```python
from build123d import *

# Parameters (mm, degrees)
F0_W     = 77.216
F0_H     = 148.336
F1_DEPTH = 14.478
F2_R     = 5.08
F3_T     = -6.858
F4_R     = 5.08


with BuildPart() as f1:
    # F0 (on Top) → F1 (new body)
    with BuildSketch(Plane.XY):
        Rectangle(F0_W, F0_H)
    extrude(amount=F1_DEPTH)

    # F2
    f2_edges = [f1.edges().sort_by_distance(p)[0] for p in [
        (-38.608, 74.168, 7.239),
        (38.608, 74.168, 7.239),
        (38.608, -74.168, 7.239),
        (-38.608, -74.168, 7.239),
        (38.608, 0, 0),
    ]]
    fillet(f2_edges, radius=F2_R)

    # F3
    f3_openings = [f1.faces().sort_by_distance(p)[0] for p in [
        (0, 0, 14.478),
    ]]
    offset(amount=F3_T, openings=f3_openings)

    # F4
    f4_edges = [f1.edges().sort_by_distance(p)[0] for p in [
        (0, -67.31, 6.858),
        (31.75, 0, 6.858),
        (0, 67.31, 6.858),
        (-31.75, 0, 6.858),
    ]]
    fillet(f4_edges, radius=F4_R)


solid = f1.part
```
Read the model definition and answer for the solid it produces. Units are mm, in the model's axes. A direction names the side the tool comes from. Round coordinates to 2 decimals unless told otherwise and drop trailing zeros. Loops run counter-clockwise (first coordinate to the right, second up) from the corner with the lowest first, then second, coordinate; pieces in that order, holes last. Notation, with made-up numbers: (4, -3) -> (19, -3) arc R24 cw to (19, 20) -> close; hole circle Ø9 at (26.25, 2.25). An arc over 180 degrees is marked (long way). One line per item, written item: value.
1) Consider L1, parallel to X at y = 21, z = 12; L2, parallel to Z at x = -22.5, y = -62; L3, parallel to Y at x = -26, z = 12.5. Determine where each line is inside the solid, lowest interval first. Write a range as [from, to].
Answer list:
L1: x = [-38.61, -31.75], [31.75, 38.61]
L2: z = [0, 6.86]
L3: y = [-74.17, -67.31], [67.31, 74.17]
2) Flat-ended cylindrical pins translate along their axes: P1, Ø5, axis at x = 16, y = 32.5, coming from the -Z side; P2, Ø10, axis at x = -3, y = -9.5, coming from the +Z side. Find the tip coordinate at first contact, or state that the pin passes through.
Answer list:
P1: stops at z = 0
P2: stops at z = 6.86
3) The mould has two halves that part along X. Classify faces 1 (the face through (-37.2, -72.6, 7.3)), 2 (the face through (37.1, -72.7, 7.3)), 3 (the face through (0, 67.31, 13)): pulls with the +X half, pulls with the -X half, needs draft (parallel to the pull), parting line crosses it, or undercut.
Answer list:
face 1: pulls with the -X half
face 2: pulls with the +X half
face 3: undercut
4) A cutting plane is placed at C-C (y = 7.5). Determine the outline of the cut face in (x, z), and give its area (3 significant figures).
Answer list:
outline: (-38.61, 0) -> (33.53, 0) arc R5.08 ccw to (38.61, 5.08) -> (38.61, 14.48) -> (31.75, 14.48) -> (31.75, 11.94) arc R5.08 cw to (26.67, 6.86) -> (-26.67, 6.86) arc R5.08 cw to (-31.75, 11.94) -> (-31.75, 14.48) -> (-38.61, 14.48) -> close
area: 640 mm²
5) A cutting plane is placed at A-A (z = 9.5). Determine the outline of the cut face in (x, y), and give its area (3 significant figures).
Answer list:
outline: (-38.61, -69.09) arc R5.08 ccw to (-33.53, -74.17) -> (33.53, -74.17) arc R5.08 ccw to (38.61, -69.09) -> (38.61, 69.09) arc R5.08 ccw to (33.53, 74.17) -> (-33.53, 74.17) arc R5.08 ccw to (-38.61, 69.09) -> close; hole (-31.13, -66.69) -> (31.13, -66.69) -> (31.13, 66.69) -> (-31.13, 66.69) -> close
area: 3,130 mm²
6) A cutting plane is placed at B-B (x = 11). Determine the outline of the cut face in (y, z), and give its area (3 significant figures).
Answer list:
outline: (-74.17, 0) -> (74.17, 0) -> (74.17, 14.48) -> (67.31, 14.48) -> (67.31, 11.94) arc R5.08 cw to (62.23, 6.86) -> (-62.23, 6.86) arc R5.08 cw to (-67.31, 11.94) -> (-67.31, 14.48) -> (-74.17, 14.48) -> close
area: 1,130 mm²
7) For faces 4 (the face through (0, 74.168, 7)), 5 (the face through (31.75, -1, 13)), determine the directions among +Z, -Z, +X, -X, +Y, -Y from which every point of the face is accessible in a straight line to the end or side of a thin tool.
Answer list:
face 4: +Z, -Z, +X, -X, +Y
face 5: +Z
